Part model, mm, in its own coordinate system. Face numbers are marked on the shaded views. A direction names the side the tool comes from. Round coordinates to 2 decimals unless told otherwise and drop trailing zeros. Loops run counter-clockwise (first coordinate to the right, second up) from the corner with the lowest first, then second, coordinate; pieces in that order, holes last.
1) 3-axis set-ups, long thin cutter, end or side, ignore diameter. For the marked faces 1 and 2: which of +Z, -Z, +X, -X, +Y, -Y reach the whole face in a straight line?
2) Drop flat-ended pins along their axis: P1, Ø12, axis at x = -11, z = 380.5, coming from the +Y side; P2, Ø1, axis at x = 0, y = 182, coming from the -Z side; P3, Ø10, axis at y = 180.5, z = 389.5, coming from the +X side. Give the stop position or say it passes through.
3) Probe line 1 (X direction, y = 189.5, z = 393); line 2 (Z direction, x = 3, y = 179.75); line 3 (Z direction, x = 0.5, y = 197.5). List the from-to ranges inside material, lowest first.
4) Band-saw the part on B-B, the plane y = 197. Write the cut outline in (x, z), then the cut area to 3 significant figures.
5) Band-saw the part on A-A, the plane y = 191.5. Write the cut outline in (x, z), then the cut area to 3 significant figures.
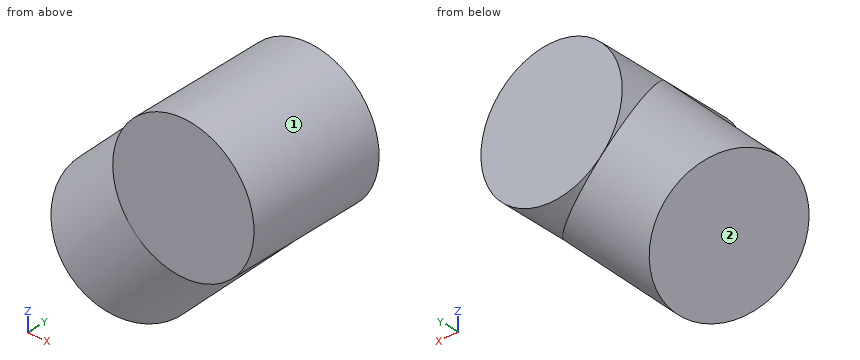
from build123d import *

# Parameters (mm, degrees)
CYLINDER046_R             = 13.9827
CYLINDER046_DEPTH         = 28.0162
CYLINDER045_R             = 13.9827
CYLINDER045_DEPTH         = 32.1945
FUSION018_PLACEMENT_ANGLE = 225


with BuildPart() as cylinder046:
    # Cylinder046 → Cylinder046 (new body)
    with BuildSketch(Plane.XZ.offset(-14.0081)):
        Circle(CYLINDER046_R)
    extrude(amount=CYLINDER046_DEPTH)


with BuildPart() as middle_inner_slip_r:
    # Cylinder045 → Cylinder045 (new body)
    with BuildSketch(Plane.XY):
        Circle(CYLINDER045_R)
    extrude(amount=CYLINDER045_DEPTH)

    # Fusion018: union Cylinder046
    add(cylinder046.part)


with BuildPart() as middle_inner_slip_r_1:
    # Fusion018 placement: moved
    add(middle_inner_slip_r.part.moved(Location((0, 186, 406))).rotate(Axis((0, 186, 406), (0, 1, 0)), FUSION018_PLACEMENT_ANGLE))


solid = middle_inner_slip_r_1.part
Reported:
1. face 1: none
1. face 2: -Z, -X, +Y, -Y
2. P1: stops at y = 199.32
2. P2: stops at z = 386.51
2. P3: stops at x = 7.95
3. line 1: x = -32.15 to 6.15
3. line 2: z = 391.31 to 419.66
3. line 3: z = 392.03 to 419.97
4. outline: (-28.87, 389.34) - (-16.66, 377.13) - (-1.67, 392.12) arc R13.98 ccw (long way) to (-13.88, 404.33) - close
4. area: 945 mm2
5. outline: (-31.86, 392.33) - (-13.67, 374.14) - (5.2, 393.02) arc R13.98 ccw (long way) to (-12.98, 411.2) - close
5. area: 1,140 mm2
